Here's how the part is built. I have some questions about the finished solid (model axes, mm). Round coordinates to 2 decimals unless told otherwise and drop trailing zeros. Write each loop counter-clockwise with the first axis right and the second up, starting at its lowest first coordinate (ties: lowest second). Pieces come first, ordered by that corner, then holes. Notation, with made-up numbers: (-23, 66) - (7, 66) arc R7 cw to (7, 78) - close; hole circle Ø6 at (0, 84). An arc over 180 degrees is marked (long way). One line per item, written item: value. Start each with the question number.
Item 1: If I drill on line 1 (Y direction, x = -1.5, z = 4.25); line 2 (Y direction, x = -5, z = -3.75); line 3 (Z direction, x = 3.75, y = -11), over which ranges is the centre line in solid material (lowest first)?
Item 2: Thinking about a two-plate mould opening in X: for faces 1 (the face through (0, 3.81, 0)), 2 (the face through (-3.86, -20.91, -5.04)), 3 (the face through (6, 0, 3)), which applies, released by +X, released by -X, zero draft, split by the parting line, or undercut?
Item 3: For P1, Ø0.8, axis at x = 0.5, z = -5.5, coming from the +Y side; P2, Ø1, axis at y = -27, z = -2.5, coming from the +X side; P3, Ø2, axis at x = 5.5, y = -3, coming from the -Z side; P4, Ø12, axis at x = 6, z = -1.5, coming from the +Y side, each with a flat end and sliding along its axis, tell me the tip position at first contact or that it passes through.
Item 4: Imagine slicing it at A-A, the plane y = -31.5. Please give me the cut outline in (x, z), then the cut area to 3 significant figures.
```python
from build123d import *

# Parameters (mm, degrees)
SKETCH1_R           = 6.35
BOSS_EXTRUDE1_DEPTH = 43.18
SKETCH1_3_R         = 12.7
BOSS_EXTRUDE2_DEPTH = 7.62
SKETCH4_W           = 2.54
SKETCH4_H           = 33.82833048
CUT_EXTRUDE1_DEPTH  = 51.305467944
CUT_EXTRUDE1_TAPER  = -30
CHAMFER1_SIZE       = 0.762


with BuildPart() as part:
    # Sketch1 → Boss-Extrude1 (new body)
    with BuildSketch(Plane(origin=(0, 0, 0), x_dir=(1, 0, 0), z_dir=(0, 1, 0))):
        with Locations(Location((0, 0, 0), (0, 0, 270))):
            Circle(SKETCH1_R)
    extrude(amount=-BOSS_EXTRUDE1_DEPTH)

    # Sketch1<3> → Boss-Extrude2 (add)
    with BuildSketch(Plane(origin=(0, 0, 0), x_dir=(1, 0, 0), z_dir=(0, 1, 0))):
        with Locations(Location((0, 0, 0), (0, 0, 270))):
            Circle(SKETCH1_3_R)
    extrude(amount=BOSS_EXTRUDE2_DEPTH)

    # Sketch3 → Cut-Revolve1 (revolve, cut)
    with BuildSketch(Plane.XY, mode=Mode.PRIVATE) as cut_revolve1_sk:
        with BuildLine():
            Line((-12.7, 2.54), (-15.209374463, 2.54))
            Line((-15.209374463, 2.54), (-15.209374463, 10.331344658))
            Line((-15.209374463, 10.331344658), (0, 10.331344658))
            Line((0, 10.331344658), (0, 7.62))
            ThreePointArc((0, 7.62), (-6.858056154, 6.350140386), (-12.7, 2.54))
        make_face()
    revolve(cut_revolve1_sk.sketch.rotate(Axis((0, 0, 0), (0, 1, 0)), 270), axis=Axis((0, 0, 0), (0, 1, 0)), mode=Mode.SUBTRACT)

    # Sketch4 → Cut-Extrude1 (cut, through all)
    with BuildSketch(Plane(origin=(0, 3.81, 0), x_dir=(1, 0, 0), z_dir=(0, 1, 0))):
        Rectangle(SKETCH4_W, SKETCH4_H)
    extrude(amount=CUT_EXTRUDE1_DEPTH, taper=CUT_EXTRUDE1_TAPER, mode=Mode.SUBTRACT)

    # Chamfer1
    chamfer1_edges = [part.edges().sort_by_distance(p)[0] for p in [
        (0, -43.18, -6.35),
    ]]
    chamfer(chamfer1_edges, length=CHAMFER1_SIZE)


solid = part.part
```
Values follow:
1. line 1: y = -43.18 to 4.21
1. line 2: y = -42.52 to 6.58
1. line 3: z = -5.12 to 5.12
2. face 1: undercut
2. face 2: split by the parting line
2. face 3: zero draft
3. P1: stops at y = 3.81
3. P2: stops at x = 6.03
3. P3: stops at z = -4.48
3. P4: stops at y = 7.36
4. outline: circle Ø12.7 at (0, 0)
4. area: 127 mm^2
